Geometry: final body of the model. Coordinates: model frame, mm. Face numbers are marked on the shaded views. A direction names the side the tool comes from. Round coordinates to 2 decimals unless told otherwise and drop trailing zeros. Loops run counter-clockwise (first coordinate to the right, second up) from the corner with the lowest first, then second, coordinate; pieces in that order, holes last. Notation, with made-up numbers: (24.25, 17) -> (75.25, 17) arc R28 ccw to (75.25, 38) -> close; hole circle Ø1 at (88.25, 25). An arc over 180 degrees is marked (long way). Answer in a Markdown table with one row per item.
```python
from build123d import *

# Parameters (mm, degrees)
CROQUIS3_R              = 15.5
CROQUIS3_R_2            = 9.5
SALIENTE_EXTRUIR3_DEPTH = 1.5
CROQUIS4_R              = 12.95
CROQUIS4_R_2            = 12.15
SALIENTE_EXTRUIR4_DEPTH = 7.3


with BuildPart() as part:
    # Croquis3 → Saliente-Extruir3 (new body)
    with BuildSketch(Plane.XY):
        with Locations((38, 0)):
            Circle(CROQUIS3_R)
        with Locations((38, 0)):
            Circle(CROQUIS3_R_2, mode=Mode.SUBTRACT)
    extrude(amount=SALIENTE_EXTRUIR3_DEPTH)

    # Croquis4 → Saliente-Extruir4 (add)
    with BuildSketch(Plane.XY.offset(1.5)):
        with Locations((38, 0)):
            Circle(CROQUIS4_R)
        with Locations((38, 0)):
            Circle(CROQUIS4_R_2, mode=Mode.SUBTRACT)
    extrude(amount=SALIENTE_EXTRUIR4_DEPTH)


solid = part.part
```
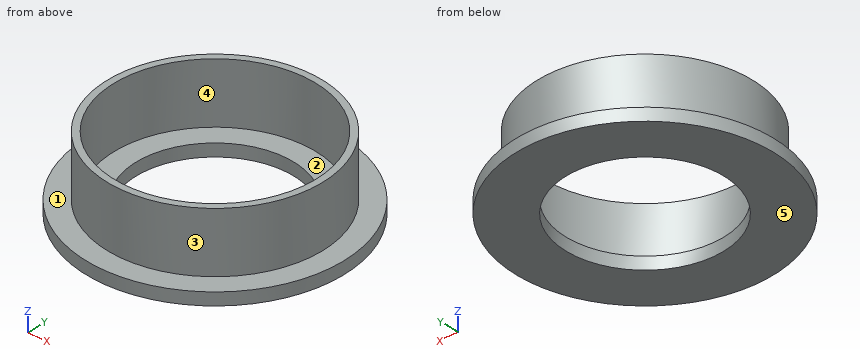
Item 1: Ray query, L1, parallel to Y at x = 38, z = 4.5; L2, parallel to Z at x = 47, y = -11.5; L3, parallel to Y at x = 31, z = 6.75. Return the intervals inside material, ascending.
Ans:
| item | result |
|---|---|
| L1 | -12.95 to -12.15, 12.15 to 12.95 |
| L2 | 0 to 1.5 |
| L3 | -10.9 to -9.93, 9.93 to 10.9 |
Item 2: First-contact query: P1, Ø7.5, axis at x = 42, y = 2.5, coming from the +Z side; P2, Ø3, axis at x = 27.5, z = 7.5, coming from the -Y side; P3, Ø2, axis at x = 32.5, z = 5, coming from the +Y side. Flat tips, straight axial feed; report the tip coordinate or a pass-through.
Ans:
| item | result |
|---|---|
| P1 | through |
| P2 | y = -9.31 |
| P3 | y = 12.14 |
Item 3: Set-up query: the marked faces 4 and 5. Return all of +Z, -Z, +X, -X, +Y, -Y with unobstructed straight access to the full face (end or side cutting, diameter ignored); none if empty.
Ans:
| item | result |
|---|---|
| face 4 | +Z |
| face 5 | -Z, +X, -X, +Y, -Y |
Item 4: Section query B-B, the plane x = 38. Output: boundary loops of the cut face in (y, z).
Ans:
| item | result |
|---|---|
| outline | (-15.5, 0) -> (-9.5, 0) -> (-9.5, 1.5) -> (-12.15, 1.5) -> (-12.15, 8.8) -> (-12.95, 8.8) -> (-12.95, 1.5) -> (-15.5, 1.5) -> close; (9.5, 0) -> (15.5, 0) -> (15.5, 1.5) -> (12.95, 1.5) -> (12.95, 8.8) -> (12.15, 8.8) -> (12.15, 1.5) -> (9.5, 1.5) -> close |
Item 5: Section query D-D, the plane y = 11.5. Output: boundary loops of the cut face in (x, z).
Ans:
| item | result |
|---|---|
| outline | (27.61, 0) -> (48.39, 0) -> (48.39, 1.5) -> (43.95, 1.5) -> (43.95, 8.8) -> (41.92, 8.8) -> (41.92, 1.5) -> (34.08, 1.5) -> (34.08, 8.8) -> (32.05, 8.8) -> (32.05, 1.5) -> (27.61, 1.5) -> close |
Item 6: Mould query, pull axis Y, two halves, no side actions, for the marked faces 1, 2 and 3. Classes: released by +Y, released by -Y, zero draft, split by the parting line, or undercut.
Ans:
| item | result |
|---|---|
| face 1 | zero draft |
| face 2 | undercut |
| face 3 | split by the parting line |
Item 7: Section query A-A, the plane y = 0. Output: boundary loops of the cut face in (x, z), and give its area (3 significant figures).
Ans:
| item | result |
|---|---|
| outline | (22.5, 0) -> (28.5, 0) -> (28.5, 1.5) -> (25.85, 1.5) -> (25.85, 8.8) -> (25.05, 8.8) -> (25.05, 1.5) -> (22.5, 1.5) -> close; (47.5, 0) -> (53.5, 0) -> (53.5, 1.5) -> (50.95, 1.5) -> (50.95, 8.8) -> (50.15, 8.8) -> (50.15, 1.5) -> (47.5, 1.5) -> close |
| area | 29.7 mm2 |
Item 8: Section query C-C, the plane z = 4.75. Output: boundary loops of the cut face in (x, y), and give its area (3 significant figures).
Ans:
| item | result |
|---|---|
| outline | circle Ø25.9 at (38, 0); hole circle Ø24.3 at (38, 0) |
| area | 63.1 mm2 |
